```python
from build123d import *

# Parameters (mm, degrees)
SKETCH1_R               = 16
SKETCH1_R_2             = 3
BOSS_EXTRUDE1_DEPTH     = 25
CUT_EXTRUDE1_DEPTH      = 6.85
CUT_EXTRUDE2_REACH      = 35.719
CUT_EXTRUDE2_END_RADIUS = 16


with BuildPart() as part:
    # Sketch1 → Boss-Extrude1 (new body)
    with BuildSketch(Plane.XY):
        Circle(SKETCH1_R)
        Circle(SKETCH1_R_2, mode=Mode.SUBTRACT)
    extrude(amount=BOSS_EXTRUDE1_DEPTH)

    # Sketch2 → Cut-Extrude1 (cut, symmetric)
    with BuildSketch(Plane(origin=(0, 0, 0), x_dir=(1, 0, 0), z_dir=(0, 1, 0))):
        with BuildLine():
            Line((-12.85, -25), (-12.85, -19.5))
            ThreePointArc((-12.85, -19.5), (0, -6.65), (12.85, -19.5))
            Line((12.85, -19.5), (12.85, -25))
            Line((12.85, -25), (-12.85, -25))
        make_face()
    extrude(amount=CUT_EXTRUDE1_DEPTH, both=True, mode=Mode.SUBTRACT)

    # Cut-Extrude2: up to this cylinder (the profile starts inside it)
    cut_extrude2_end = Plane(origin=(0, 0, 20.344451), z_dir=(0, 0, -1)) * Cylinder(CUT_EXTRUDE2_END_RADIUS, 104.438, mode=Mode.PRIVATE)
    # Sketch3 → Cut-Extrude2 (cut, up to the surface)
    with BuildSketch(Plane(origin=(0, 0, 0), x_dir=(1, 0, 0), z_dir=(0, 1, 0)), mode=Mode.PRIVATE) as cut_extrude2_sk1:
        with BuildLine():
            Line((-4.7, -19.5), (-4.7, -25))
            Line((-4.7, -25), (4.7, -25))
            Line((4.7, -25), (4.7, -19.5))
            ThreePointArc((4.7, -19.5), (0, -14.8), (-4.7, -19.5))
        make_face()
    cut_extrude2_tool1 = extrude(cut_extrude2_sk1.sketch, amount=-CUT_EXTRUDE2_REACH, mode=Mode.PRIVATE) & cut_extrude2_end
    add(cut_extrude2_tool1.solids().sort_by_distance((0, 0, 20.344451))[0], mode=Mode.SUBTRACT)


solid = part.part
```
Build history of the part. All positions in model axes, mm. A direction names the side the tool comes from. Coordinates: 2 decimals unless noted, no trailing zeros. Order: outer loops, then holes, each group sorted by start corner. A loop starts at its lowest first (then second) coordinate and runs counter-clockwise, first axis right, second up. Notation, with made-up numbers: (46.25, 48.25) -> (78.25, 48.25) arc R25 cw to (78.25, 77.25) -> close; hole circle Ø9 at (72.5, 40). An arc over 180 degrees is marked (long way). Answer in a Markdown table with one row per item. Add a question column.
Q1. Band-saw the part on D-D, the plane y = -10. List the corners of the cut face in (x, z).
Q2. Drop flat-ended pins along their axis: pin 1 (1.6 mm diameter, centred on y = -11, z = 23.5, fed in from +X); pin 2 (12 mm diameter, centred on x = 5.5, y = -4, fed in from +Z); pin 3 (2 mm diameter, centred on y = -7, z = 15, fed in from +X); pin 4 (6 mm diameter, centred on x = 6, z = 8.5, fed in from +Y). Give the stop position or say it passes through.
Q3. Band-saw the part on A-A, the plane y = 0. List the corners of the cut face in (x, z), then the cut area to 3 significant figures.
Q4. Mould opens along Y. For faces 1 (the face through (0.1, -11.4, 14.8)), 2 (the face through (8.6, 13.49, 12.32)), 3 (the face through (-12.85, 0, 22)) say: +Y half, -Y half, draft (parallel to the pull), parting line (faces both ways), or undercut.
Q5. Wall check: line 1 along Y through (x, z) = (0, 4.5); line 2 along X through (y, z) = (5, 12.5). Give the ranges that are in metal, low to high. Write a range as [from, to].
Q6. Which spindle directions (+Z, -Z, +X, -X, +Y, -Y) get a long thin tool onto all of the face, cutting with end or side? Do faces 4 (the face through (-4.7, -11, 22)), 5 (the face through (-3, 0, 3)), 6 (the face through (-0.283, 3.14, 6.653)). Say none if no direction does.
Q7. Band-saw the part on C-C, the plane z = 9. List the corners of the cut face in (x, y).
Q8. Band-saw the part on B-B, the plane x = 0. List the corners of the cut face in (y, z).
Answers follow:
| question | item | result |
|---|---|---|
| 1 | outline | (-12.49, 0) -> (12.49, 0) -> (12.49, 25) -> (4.7, 25) -> (4.7, 19.5) arc R4.7 cw to (-4.7, 19.5) -> (-4.7, 25) -> (-12.49, 25) -> close |
| 2 | pin 1 | x = 12.33 |
| 2 | pin 2 | z = 25 |
| 2 | pin 3 | x = 14.83 |
| 2 | pin 4 | y = 15.72 |
| 3 | outline | (-16, 0) -> (-3, 0) -> (-3, 7.01) arc R12.85 cw to (-12.85, 19.5) -> (-12.85, 25) -> (-16, 25) -> close; (3, 0) -> (16, 0) -> (16, 25) -> (12.85, 25) -> (12.85, 19.5) arc R12.85 cw to (3, 7.01) -> close |
| 3 | area | 359 mm^2 |
| 4 | face 1 | draft |
| 4 | face 2 | parting line |
| 4 | face 3 | undercut |
| 5 | line 1 | [-16, -3], [3, 16] |
| 5 | line 2 | [-15.2, -10.78], [10.78, 15.2] |
| 6 | face 4 | +Z, -Y |
| 6 | face 5 | +Z, -Z |
| 6 | face 6 | +Z |
| 7 | outline | circle Ø32 at (0, 0); hole (-7.41, -6.85) -> (7.41, -6.85) -> (7.41, 6.85) -> (-7.41, 6.85) -> close |
| 8 | outline | (-16, 0) -> (-3, 0) -> (-3, 6.65) -> (-6.85, 6.65) -> (-6.85, 14.8) -> (-16, 14.8) -> close; (3, 0) -> (16, 0) -> (16, 25) -> (6.85, 25) -> (6.85, 6.65) -> (3, 6.65) -> close |
